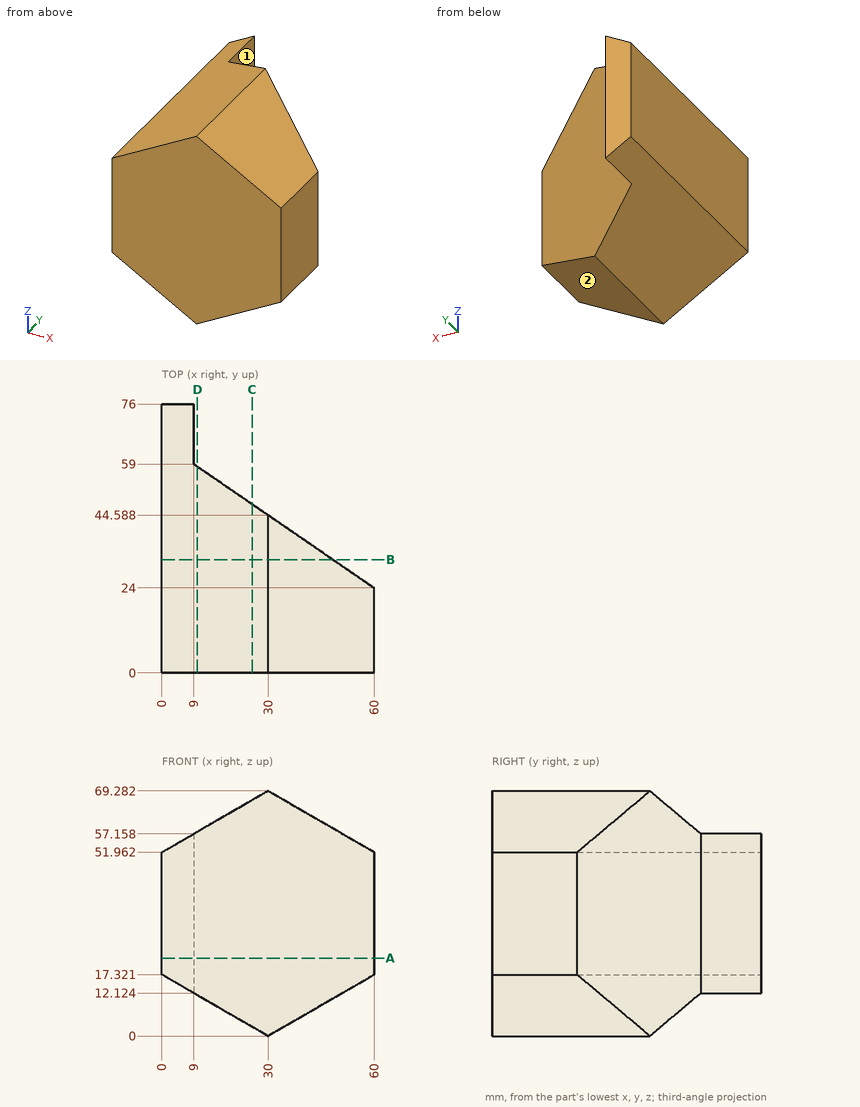
Study the drawing (mm; zero at the part's minimum x, y, z) and answer. A direction names the side the tool comes from. Give positions to 0.01 mm unless a question says otherwise; leave off trailing zeros. Write each loop counter-clockwise with the first axis right and the second up, starting at its lowest first coordinate (ties: lowest second). Pieces come first, ordered by that corner, then holes. Notation, with made-up numbers: M 6.25,-24 L 58.25,-24 A14 ccw 58.25,-19 Z; hole C -21.75,42 d9. An arc over 180 degrees is marked long. Put each result on its own line as item: value. Start each with the question number.
1. The part is cut by section C-C, the plane x = 25.5. Give the vertices of the cut face in (y, z), and give its area (3 significant figures).
2. The part is cut by section A-A, the plane z = 22. Give the vertices of the cut face in (x, y), and give its area (3 significant figures).
3. Which of the six approach directions +Z, -Z, +X, -X, +Y, -Y give full straight-line access (tool end or side, diameter ignored) to the marked faces 1 and 2?
4. The part is cut by section B-B, the plane y = 32. Give the vertices of the cut face in (x, z), and give its area (3 significant figures).
5. The part is cut by section D-D, the plane x = 10. Give the vertices of the cut face in (y, z) (1 decimal).
6. Consider line 1 along X through (y, z) = (73, 20); line 2 along X through (y, z) = (72.5, 16.5) (1 decimal); line 3 along Y through (x, z) = (50, 48) (1 decimal). Determine where each line is inside the solid, lowest interval first.
7. Each of these flat-tipped pins is pushed along its axis until it touches: pin 1 Ø3 at (x, z) = (31.5, 35) entering from -Y; pin 2 Ø1 at (y, z) = (44, 60) entering from +X (1 decimal); pin 3 Ø1 at (y, z) = (40.5, 50.5) entering from +X (1 decimal); pin 4 Ø12 at (x, y) = (8, 26) entering from -Z. Where does it stop, or does it pass through?
Final values:
1. outline: M 0,2.6 L 47.68,2.6 L 47.68,66.68 L 0,66.68 Z
1. area: 3,060 mm²
2. outline: M 0,0 L 60,0 L 60,24 L 9,59 L 9,76 L 0,76 Z
2. area: 2,800 mm²
3. face 1: +Z, -Z, +X, +Y
3. face 2: -Z, +X, +Y, -Y
4. outline: M 0,17.32 L 30,0 L 48.34,10.59 L 48.34,58.69 L 30,69.28 L 0,51.96 Z
4. area: 2,640 mm²
5. outline: M 0,11.5 L 58.3,11.5 L 58.3,57.7 L 0,57.7 Z
6. line 1: x = 0 to 9
6. line 2: x = 1.4 to 9
6. line 3: y = 0 to 30.9
7. pin 1: stops at y = 0
7. pin 2: stops at x = 31.6
7. pin 3: stops at x = 36.7
7. pin 4: stops at z = 9.24
